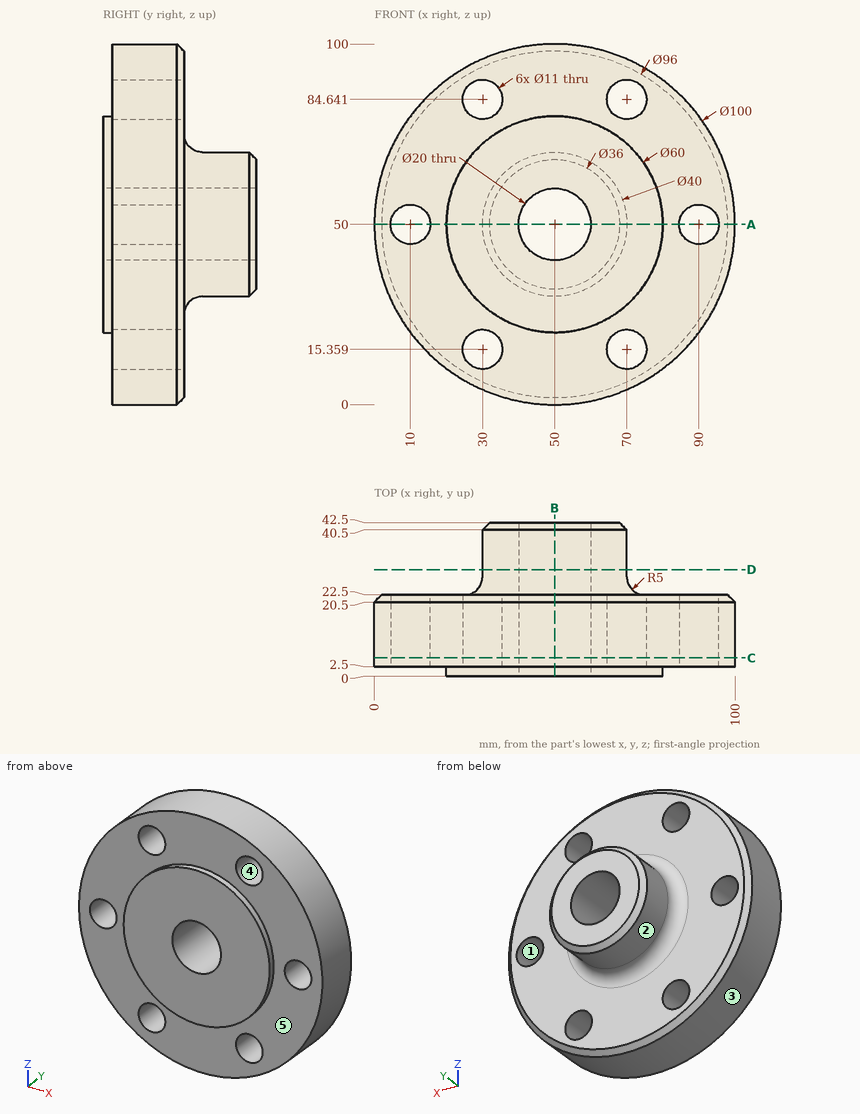
Study the drawing (mm; zero at the part's minimum x, y, z) and answer. A direction names the side the tool comes from. Coordinates: 2 decimals unless noted, no trailing zeros. Loops run counter-clockwise (first coordinate to the right, second up) from the corner with the lowest first, then second, coordinate; pieces in that order, holes last. Notation, with made-up numbers: M -10.5,53.25 L 37.5,53.25 A20 cw 37.5,68.25 Z; hole C 40.25,10 d10. An arc over 180 degrees is marked long. Answer as a JSON object with one key per item and string values. Group by question number.
Item 1: Which of the six approach directions +Z, -Z, +X, -X, +Y, -Y give full straight-line access (tool end or side, diameter ignored) to the marked faces 1 and 2?
Item 2: Section D-D (y = 29.5) is taken. Write down the section's boundary in (x, z).
Item 3: Section A-A (z = 50) is taken. Give the number of separate pieces and of enclosed holes in the cut face, and give its area (3 significant figures).
Item 4: Section C-C (y = 5) is taken. Write down the section's boundary in (x, z).
Item 5: Section B-B (x = 50) is taken. Write down the section's boundary in (y, z), and give its area (3 significant figures).
Item 6: Determine the mould class of the marked faces 3, 4 and 5 for opening direction Z: +Z half, -Z half, draft (parallel to the pull), parting line (faces both ways), or undercut.
Item 7: Each of these flat-tipped pins is pushed along its axis until it touches: P1, Ø12.5, axis at x = 30, z = 15.36, coming from the +Y side; P2, Ø1, axis at x = 69, y = 17, coming from the -Z side; P3, Ø17.5, axis at x = 70, z = 15.36, coming from the -Y side. Where does it stop, or does it pass through?
Item 8: Consider L1, parallel to Z at x = 30, y = 7; L2, parallel to Y at x = 25, z = 41.5; L3, parallel to Y at x = 54, z = 5. Determine where each line is inside the solid, lowest interval first.
Solved:
{
 "1": {"face 1": "+Y, -Y", "face 2": "+Y"},
 "2": {"outline": "C 50,50 d40; hole C 50,50 d20"},
 "3": {"separate pieces": "4", "enclosed holes": "0", "area": "1,660 mm2"},
 "4": {"outline": "C 50,50 d100; hole C 10,50 d11; hole C 30,15.36 d11; hole C 30,84.64 d11; hole C 50,50 d20; hole C 70,15.36 d11; hole C 70,84.64 d11; hole C 90,50 d11"},
 "5": {"outline": "M 0,20 L 2.5,20 L 2.5,0 L 20.5,0 L 22.5,2 L 22.5,25 A5 cw 27.5,30 L 40.5,30 L 42.5,32 L 42.5,40 L 0,40 Z; M 0,60 L 42.5,60 L 42.5,68 L 40.5,70 L 27.5,70 A5 cw 22.5,75 L 22.5,98 L 20.5,100 L 2.5,100 L 2.5,80 L 0,80 Z", "area": "2,100 mm2"},
 "6": {"face 3": "parting line", "face 4": "undercut", "face 5": "draft"},
 "7": {"P1": "stops at y = 22.5", "P2": "stops at z = 3.55", "P3": "stops at y = 2.5"},
 "8": {"L1": "z = 4.17 to 9.86, 20.86 to 79.14, 90.14 to 95.83", "L2": "y = 0 to 22.5", "L3": "y = 2.5 to 22.5"}
}
